Here's how the part is built. I have some questions about the finished solid (model axes, mm). Face numbers are marked on the shaded views. A direction names the side the tool comes from. Coordinates: 2 decimals unless noted, no trailing zeros. Order: outer loops, then holes, each group sorted by start corner. A loop starts at its lowest first (then second) coordinate and runs counter-clockwise, first axis right, second up.
```python
from build123d import *

# Parameters (mm, degrees)
SKETCH1_W                        = 44.45
SKETCH1_H                        = 25.4
BOSS_EXTRUDE1_DEPTH              = 12.7
CUT_EXTRUDE1_REACH               = 46.45
SKETCH2_R                        = 3.96875
F_18_0_1695_DIAMETER_HOLE1_D     = 4.3053
F_18_0_1695_DIAMETER_HOLE1_DEPTH = 12.7
SKETCH5_W                        = 44.45
SKETCH5_H                        = 13.74547341
CUT_EXTRUDE2_DEPTH               = 8.73125


with BuildPart() as part:
    # Sketch1 → Boss-Extrude1 (new body)
    with BuildSketch(Plane(origin=(0, 0, 0), x_dir=(1, 0, 0), z_dir=(0, 1, 0))):
        with Locations((-34.470243637, -32.242582921)):
            Rectangle(SKETCH1_W, SKETCH1_H)
    extrude(amount=BOSS_EXTRUDE1_DEPTH)

    # Sketch2 → Cut-Extrude1 (cut, up to next)
    with BuildSketch(Plane(origin=(-12.245243637, 0, 0), x_dir=(0, 0, -1), z_dir=(1, 0, 0)), mode=Mode.PRIVATE) as cut_extrude1_sk1:
        with Locations((-24.543510458, 6.746875)):
            Circle(SKETCH2_R)
    cut_extrude1_tool1 = extrude(cut_extrude1_sk1.sketch, amount=-CUT_EXTRUDE1_REACH, mode=Mode.PRIVATE) & part.part
    add(cut_extrude1_tool1.solids().sort_by_distance((-12.245244, 6.746875, 24.54351))[0], mode=Mode.SUBTRACT)

    # #18 (0.1695) Diameter Hole1
    with Locations(Plane(origin=(0, 12.7, 0), x_dir=(-1, 0, 0), z_dir=(0, 1, 0))):
        with Locations((50.345243637, 37.243510458), (18.595243637, 37.243510458)):
            Hole(F_18_0_1695_DIAMETER_HOLE1_D / 2, depth=F_18_0_1695_DIAMETER_HOLE1_DEPTH)

    # Sketch5 → Cut-Extrude2 (cut)
    with BuildSketch(Plane(origin=(0, 12.7, 0), x_dir=(1, 0, 0), z_dir=(0, 1, 0))):
        with Locations((-34.470243637, -38.069846216)):
            Rectangle(SKETCH5_W, SKETCH5_H)
    extrude(amount=-CUT_EXTRUDE2_DEPTH, mode=Mode.SUBTRACT)


solid = part.part
```
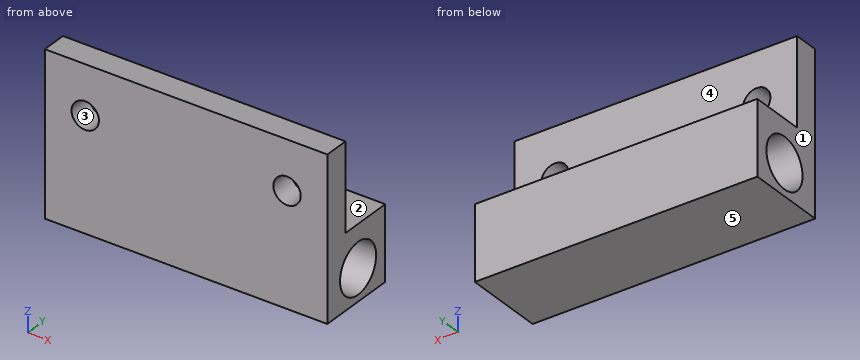
Q1. Will these pins go through, and if not, where does the flat tip stop? pin 1 (7 mm diameter, centred on x = -39, z = 36.5, fed in from +Y); pin 2 (2.5 mm diameter, centred on x = -35.5, y = 7.5, fed in from +Z); pin 3 (1 mm diameter, centred on y = 5, z = 33.5, fed in from +X).
Q2. I need wall thicknesses on L1, parallel to Y at x = -37.5, z = 33.5; L2, parallel to Z at x = -35.5, y = 9.5; L3, parallel to Z at x = -43.5, y = 4.75. Which ranges of each line are inside material? Lowest first, please.
Q3. If we section it at D-D on z = 38: Write out the boundary of the cut face in (x, y), then the cut area to 3 significant figures.
Q4. For the marked faces 4 and 5, which set-ups out of +Z, -Z, +X, -X, +Y, -Y let a thin tool reach every point of the face, with its end or its side?
Q5. If we section it at B-B on z = 25.25: Write out the boundary of the cut face in (x, y).
Q6. If we section it at A-A on x = -51.5: Write out the boundary of the cut face in (y, z).
Q7. We'd pull the mould along X, two halves only. Please class the marked faces 1, 2 and 3: pulls with the +X half, pulls with the -X half, needs draft (parallel to the pull), parting line crosses it, or undercut.
Q8. If we section it at C-C on y = 5: Write out the boundary of the cut face in (x, z), then the cut area to 3 significant figures.
Reply:
1. pin 1: stops at y = 3.97
1. pin 2: stops at z = 31.2
1. pin 3: passes through
2. L1: y = 0 to 3.97
2. L2: z = 19.54 to 21.68, 27.4 to 31.2
2. L3: z = 19.54 to 21.11, 27.97 to 31.2
3. outline: (-56.7, 0) - (-52.36, 0) - (-52.36, 3.97) - (-56.7, 3.97) - close; (-48.33, 0) - (-20.61, 0) - (-20.61, 3.97) - (-48.33, 3.97) - close; (-16.58, 0) - (-12.25, 0) - (-12.25, 3.97) - (-16.58, 3.97) - close
3. area: 144 mm2
4. face 4: +Z, +X, -X, +Y
4. face 5: -Z, +X, -X, +Y, -Y
5. outline: (-56.7, 0) - (-12.25, 0) - (-12.25, 2.84) - (-56.7, 2.84) - close; (-56.7, 10.65) - (-12.25, 10.65) - (-12.25, 12.7) - (-56.7, 12.7) - close
6. outline: (0, 19.54) - (12.7, 19.54) - (12.7, 31.2) - (3.97, 31.2) - (3.97, 35.43) - (0, 35.43) - close; (0, 39.06) - (3.97, 39.06) - (3.97, 44.94) - (0, 44.94) - close; hole circle Ø7.94 at (6.75, 24.54)
7. face 1: pulls with the -X half
7. face 2: needs draft
7. face 3: undercut
8. outline: (-56.7, 19.54) - (-12.25, 19.54) - (-12.25, 20.98) - (-56.7, 20.98) - close; (-56.7, 28.11) - (-12.25, 28.11) - (-12.25, 31.2) - (-56.7, 31.2) - close
8. area: 201 mm2
